For this review, use the dimensioned drawing (mm, ordinates from the lowest corner) and the shaded views. A direction names the side the tool comes from. Round coordinates to 2 decimals unless told otherwise and drop trailing zeros. Write each loop counter-clockwise with the first axis right and the second up, starting at its lowest first coordinate (ties: lowest second). Pieces come first, ordered by that corner, then holes. Notation, with made-up numbers: M -28,46.5 L 24,46.5 A3 ccw 24,51.5 Z; hole C 89,42 d4. An arc over 180 degrees is marked long. Use one line per item in the form item = value. Start each with the question number.
Item 1: For P1, Ø3, axis at x = 36, y = 3, coming from the -Z side; P2, Ø1, axis at y = 8.5, z = 22.5, coming from the +X side; P3, Ø3.5, axis at x = 52, y = 14, coming from the +Z side, all flat-tipped, find the tip position at first contact; note any pin that passes through.
Item 2: For line 1 (X direction, y = 13.5, z = 33.5) (1 decimal); line 2 (Z direction, x = 31.5, y = 1); line 3 (X direction, y = 6, z = 15.5) (1 decimal), list the stretches that pass through material, from the lowest coordinate up. Write a range as [from, to].
Item 3: Add section D-D (x = 49). State the section outline as (y, z) points (1 decimal).
Item 4: Add section A-A (x = 17). State the section outline as (y, z) points (1 decimal).
Item 5: For the marked faces 1, 2, 3, 4 and 5, list the 3-axis set-ups (+Z, -Z, +X, -X, +Y, -Y) from which the entire face can be reached by the end or side of a thin tool; tool diameter is ignored.
Item 6: Add section C-C (z = 37). State the section outline as (x, y) points (1 decimal).
Item 7: Add section B-B (y = 1.5). State the section outline as (x, z) points (1 decimal).
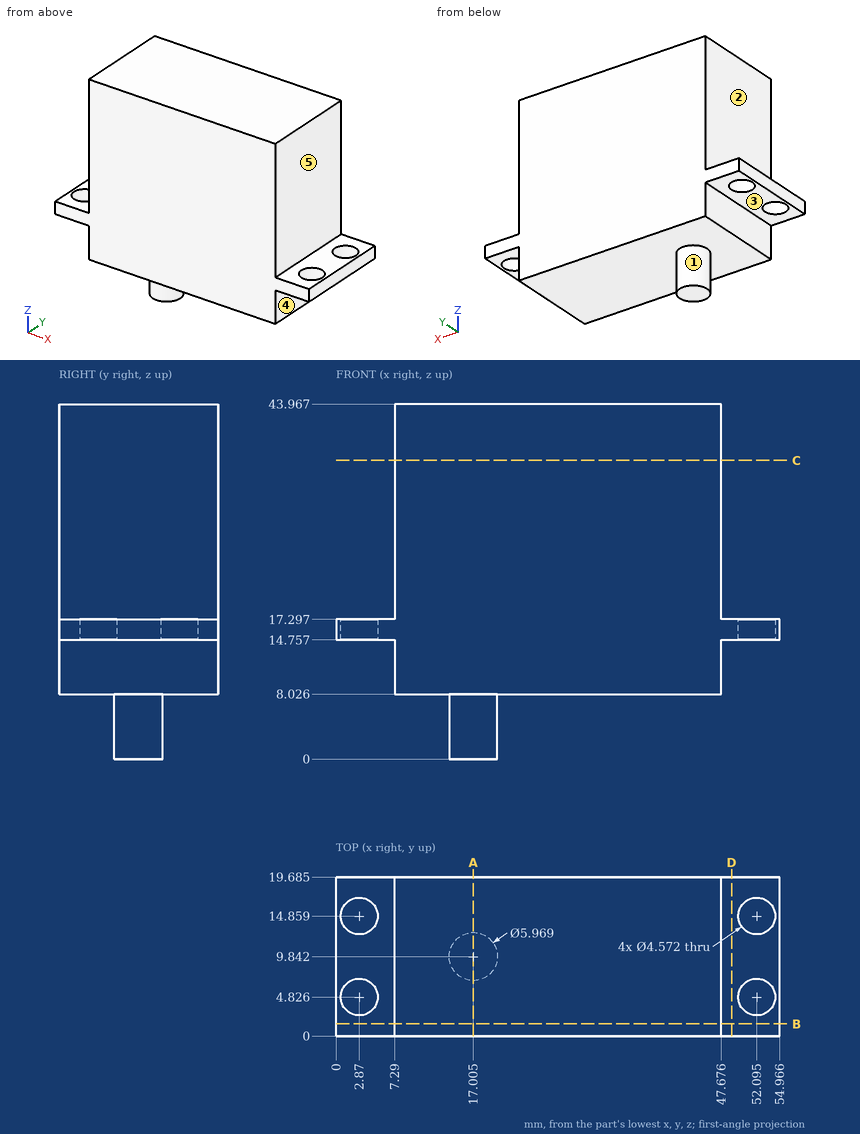
Calculated:
q1.P1 = 8.03
q1.P2 = 47.68
q1.P3 = 17.3
q2.line_1 = [7.3, 47.7]
q2.line_2 = [8.03, 43.97]
q2.line_3 = [0, 0.9], [4.8, 50.1], [54.1, 55]
q3.outline = M 0,14.8 L 19.7,14.8 L 19.7,17.3 L 0,17.3 Z
q4.outline = M 0,8 L 6.9,8 L 6.9,0 L 12.8,0 L 12.8,8 L 19.7,8 L 19.7,44 L 0,44 Z
q5.face_1 = -Z
q5.face_2 = +Z, -X, +Y, -Y
q5.face_3 = -Z, -X, +Y, -Y
q5.face_4 = -Z, +X, +Y, -Y
q5.face_5 = +Z, +X, +Y, -Y
q6.outline = M 7.3,0 L 47.7,0 L 47.7,19.7 L 7.3,19.7 Z
q7.outline = M 0,14.8 L 7.3,14.8 L 7.3,8 L 47.7,8 L 47.7,14.8 L 55,14.8 L 55,17.3 L 47.7,17.3 L 47.7,44 L 7.3,44 L 7.3,17.3 L 0,17.3 Z
